```python
from build123d import *

# Parameters (mm, degrees)
BOSS_EXTRUDE1_DEPTH   = 18
F_8_0MM_DOWEL_HOLE1_D = 9
CUT_EXTRUDE3_DEPTH    = 35
CUT_EXTRUDE4_DEPTH    = 3


with BuildPart() as part:
    # Sketch1 → Boss-Extrude1 (new body, symmetric)
    with BuildSketch(Plane.XY):
        with BuildLine():
            Line((-18.027756377, 6), (-22, 6))
            Line((-22, 6), (-22, 19))
            Line((-22, 19), (-50, 19))
            Line((-50, 19), (-50, 28))
            Line((-50, 28), (-25.690465157, 28))
            ThreePointArc((-25.690465157, 28), (0, 38), (25.690465157, 28))
            Line((25.690465157, 28), (50, 28))
            Line((50, 28), (50, 19))
            Line((50, 19), (22, 19))
            Line((22, 19), (22, 6))
            Line((22, 6), (18.027756377, 6))
            ThreePointArc((18.027756377, 6), (0, 19), (-18.027756377, 6))
        make_face()
    extrude(amount=BOSS_EXTRUDE1_DEPTH, both=True)

    # Ø8.0mm Dowel Hole1 (through all)
    with Locations(Plane(origin=(0, 28, 0), x_dir=(1, 0, 0), z_dir=(0, 1, 0))):
        with Locations((-31, 0)):
            f_8_0mm_dowel_hole1 = Hole(F_8_0MM_DOWEL_HOLE1_D / 2)

    # Sketch6 → Cut-Extrude3 (cut)
    with BuildSketch(Plane(origin=(0, 28, 0), x_dir=(1, 0, 0), z_dir=(0, 1, 0))):
        with BuildLine():
            Line((-44.497190923, 18), (-50, 18))
            Line((-50, 18), (-50, -18))
            Line((-50, -18), (-44.497190923, -18))
            ThreePointArc((-44.497190923, -18), (-48, 0), (-44.497190923, 18))
        make_face()
        with BuildLine():
            Line((44.497190923, 18), (50, 18))
            Line((50, 18), (50, -18))
            Line((50, -18), (44.497190923, -18))
            ThreePointArc((44.497190923, -18), (48, 0), (44.497190923, 18))
        make_face()
    extrude(amount=-CUT_EXTRUDE3_DEPTH, mode=Mode.SUBTRACT)

    # Sketch9 → Cut-Extrude4 (cut)
    with BuildSketch(Plane(origin=(0, 28, 0), x_dir=(1, 0, 0), z_dir=(0, 1, 0))):
        with BuildLine():
            Line((-25.690465157, 6.637683312), (-25.690465157, -6.637683312))
            ThreePointArc((-25.690465157, -6.637683312), (-22.5, 0), (-25.690465157, 6.637683312))
        make_face()
    cut_extrude4 = extrude(amount=CUT_EXTRUDE4_DEPTH, mode=Mode.SUBTRACT)

    # Mirror3: Cut-Extrude4 across plane
    add(cut_extrude4.mirror(Plane(origin=(0, 0, 0), x_dir=(0, 0, 1), z_dir=(1, 0, 0))), mode=Mode.SUBTRACT)

    # Mirror4: Ø8.0mm Dowel Hole1 across plane
    add(f_8_0mm_dowel_hole1.mirror(Plane(origin=(0, 0, 0), x_dir=(0, 0, 1), z_dir=(1, 0, 0))), mode=Mode.SUBTRACT)

    # Sketch10 → CBORE for M5 Hex Head Bolt2 (revolve, cut)
    with BuildSketch(Plane(origin=(-0.090113613, 37.999893152, -0.630795288), x_dir=(-0.999997188, -0.002371411, 0), z_dir=(0, 0, 1))):
        Polygon((0, 0), (0, 32.113844592), (2.5, 32.113844592), (2.5, 13.300129879), (2.9995, 13), (3, 0), align=None)
    revolve(axis=Axis((-0.105172072, 44.349875297, -0.630795288), (0.002371411, -0.999997188, 0)), mode=Mode.SUBTRACT)


solid = part.part
```
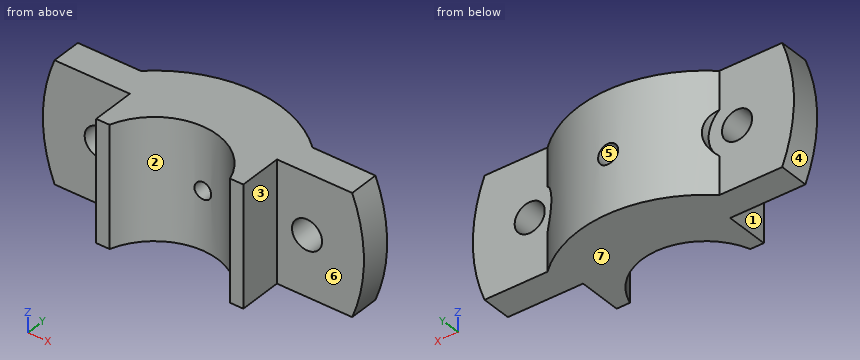
Could you check a few things on this model? Use its own coordinates, in mm. Face numbers are marked on the shaded views. A direction names the side the tool comes from. Coordinates: 2 decimals unless noted, no trailing zeros. Order: outer loops, then holes, each group sorted by start corner. A loop starts at its lowest first (then second) coordinate and runs counter-clockwise, first axis right, second up. Notation, with made-up numbers: M 18,-32 L 46,-32 A13 ccw 46,-8 Z; hole C 16.5,-14.5 d3. An arc over 180 degrees is marked long. Use one line per item in the form item = value. Start each with the question number.
1. Suppose I cut it at A-A on x = -31. Write out the boundary of the cut face in (y, z).
2. We'd pull the mould along Z, two halves only. Please class the marked faces 4, 5, 6 and 7: +Z half, -Z half, draft (parallel to the pull), parting line (faces both ways), or undercut.
3. Suppose I cut it at B-B on y = 8.5. Write out the boundary of the cut face in (x, z), then the cut area to 3 significant figures.
4. Please list where these lines run through material, in increasing order: line 1 (Z direction, x = 31, y = 24); line 2 (Y direction, x = -43, z = -10.5); line 3 (X direction, y = 14.5, z = 0.5).
5. On a 3-axis mill with a long thin cutter (end or side, diameter ignored), from which of +Z, -Z, +X, -X, +Y, -Y can I reach the whole of each face in a straight line? I mean the marked faces 1, 2 and 3. Say none if no direction works.
6. Suppose I cut it at D-D on x = 38.5. Write out the boundary of the cut face in (y, z), then the cut area to 3 significant figures.
7. Suppose I cut it at C-C on z = 14.5. Write out the boundary of the cut face in (x, y).
8. For pin 1 (10.5 mm diameter, centred on y = 11.5, z = -4.5, fed in from +X); pin 2 (2 mm diameter, centred on y = 30.5, z = 11.5, fed in from -X); pin 3 (11.5 mm diameter, centred on x = -31, z = 0, fed in from -Y); pin 4 (8 mm diameter, centred on x = 31, z = 0, fed in from -Y), each with a flat end and sliding along its axis, tell me the tip position at first contact or that it passes through.
Geometry says:
q1.outline = M 19,-18 L 28,-18 L 28,-4.5 L 19,-4.5 Z; M 19,4.5 L 28,4.5 L 28,18 L 19,18 Z
q2.face_4 = parting line
q2.face_5 = undercut
q2.face_6 = draft
q2.face_7 = -Z half
q3.outline = M -22,-18 L -16.99,-18 L -16.99,18 L -22,18 Z; M 16.99,-18 L 22,-18 L 22,18 L 16.99,18 Z
q3.area = 361 mm^2
q4.line_1 = -18 to -4.5, 4.5 to 18
q4.line_2 = 19 to 28
q4.line_3 = -22 to -12.28, 12.28 to 22
q5.face_1 = +Z, -Z, -X, -Y
q5.face_2 = +Z, -Z, -Y
q5.face_3 = +Z, -Z, +X, -Y
q6.outline = M 19,-18 L 28,-18 L 28,18 L 19,18 Z
q6.area = 324 mm^2
q7.outline = M -45.76,19 L -22,19 L -22,6 L -18.03,6 A19 cw 18.03,6 L 22,6 L 22,19 L 45.76,19 L 45.76,28 L 25.69,28 A38 ccw -25.69,28 L -45.76,28 Z
q8.pin_1 = 22
q8.pin_2 = -23.95
q8.pin_3 = 19
q8.pin_4 = through
